```python
from build123d import *

# Parameters (mm, degrees)
SKETCH1_W           = 20
SKETCH1_H           = 20
SKETCH1_R           = 1.55
BOSS_EXTRUDE1_DEPTH = 40
SKETCH2_R           = 3.75
SKETCH2_R_2         = 1.55
BOSS_EXTRUDE2_DEPTH = 40


with BuildPart() as part:
    # Sketch1 → Boss-Extrude1 (new body)
    with BuildSketch(Plane.XY):
        Rectangle(SKETCH1_W, SKETCH1_H)
        Circle(SKETCH1_R, mode=Mode.SUBTRACT)
    extrude(amount=BOSS_EXTRUDE1_DEPTH)

    # Sketch2 → Boss-Extrude2 (add)
    with BuildSketch(Plane.XY.offset(40)):
        with Locations(Location((0, 0, 0), (0, 0, 180))):
            Circle(SKETCH2_R)
        Circle(SKETCH2_R_2, mode=Mode.SUBTRACT)
    extrude(amount=BOSS_EXTRUDE2_DEPTH)


solid = part.part
```
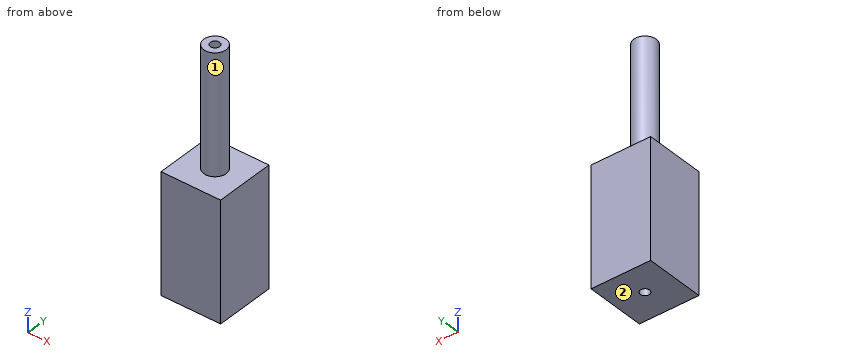
Model file for the job. Use its own axes, mm. Face numbers are marked on the shaded views. A direction names the side the tool comes from. Coordinates: 2 decimals unless noted, no trailing zeros. Order: outer loops, then holes, each group sorted by start corner. A loop starts at its lowest first (then second) coordinate and runs counter-clockwise, first axis right, second up. Notation, with made-up numbers: (-28.75, -19) -> (12.25, -19) arc R17 ccw to (12.25, -7) -> close; hole circle Ø7 at (23.25, 47). An arc over 180 degrees is marked (long way). Answer as a JSON object with one key per item and string values. Group by question number.
1) Cut at D-D, the plane x = -7.25. Write the cut outline in (y, z).
2) Which spindle directions (+Z, -Z, +X, -X, +Y, -Y) get a long thin tool onto all of the face, cutting with end or side? Do the marked faces 1 and 2. Say none if no direction does.
3) Cut at C-C, the plane z = 26. Write the cut outline in (x, y).
4) Cut at A-A, the plane x = 0. Write the cut outline in (y, z), then the cut area to 3 significant figures.
5) Flat gauge pins, fed straight in: pin 1 (1.9 mm diameter, centred on x = 0, y = 0, fed in from -Z); pin 2 (8 mm diameter, centred on y = -3, z = 71.5, fed in from +X). Where does each tip first touch, or does it go through?
6) Drill centre lines: L1, parallel to Y at x = 0, z = 27; L2, parallel to Z at x = -4.75, y = 1.25; L3, parallel to Y at x = 0, z = 54. Where is each one in solid material? Low to high.
Check values:
{
 "1": {"outline": "(-10, 0) -> (10, 0) -> (10, 40) -> (-10, 40) -> close"},
 "2": {"face 1": "+Z", "face 2": "-Z, +X, -X, +Y, -Y"},
 "3": {"outline": "(-10, -10) -> (10, -10) -> (10, 10) -> (-10, 10) -> close; hole circle Ø3.1 at (0, 0)"},
 "4": {"outline": "(-10, 0) -> (-1.55, 0) -> (-1.55, 80) -> (-3.75, 80) -> (-3.75, 40) -> (-10, 40) -> close; (1.55, 0) -> (10, 0) -> (10, 40) -> (3.75, 40) -> (3.75, 80) -> (1.55, 80) -> close", "area": "852 mm²"},
 "5": {"pin 1": "passes through", "pin 2": "stops at x = 3.75"},
 "6": {"L1": "y = -10 to -1.55, 1.55 to 10", "L2": "z = 0 to 40", "L3": "y = -3.75 to -1.55, 1.55 to 3.75"}
}
